```python
from build123d import *

# Parameters (mm, degrees)
BOSS_EXTRUDE1_DEPTH = 12.7
SKETCH2_R           = 3.175
CUT_EXTRUDE1_DEPTH  = 223.159267194


with BuildPart() as part:
    # Sketch1 → Boss-Extrude1 (new body)
    with BuildSketch(Plane(origin=(0, 0, 0), x_dir=(1, 0, 0), z_dir=(0, 1, 0))):
        with BuildLine():
            Line((-88.9, -25.4), (-71.842048969, -25.4))
            ThreePointArc((-71.842048969, -25.4), (0, -76.2), (71.842048969, -25.4))
            Line((71.842048969, -25.4), (88.9, -25.4))
            Line((88.9, -25.4), (88.9, -203.2))
            Line((88.9, -203.2), (-88.9, -203.2))
            Line((-88.9, -203.2), (-88.9, -25.4))
        make_face()
    extrude(amount=BOSS_EXTRUDE1_DEPTH)

    # Sketch2 → Cut-Extrude1 (cut, through all)
    with BuildSketch(Plane(origin=(0, 12.7, 0), x_dir=(1, 0, 0), z_dir=(0, 1, 0))):
        with Locations(Location((-19.05, -184.15, 0), (0, 0, 270))):
            Circle(SKETCH2_R)
        with Locations(Location((19.05, -184.15, 0), (0, 0, 270))):
            Circle(SKETCH2_R)
        with Locations(Location((57.15, -184.15, 0), (0, 0, 270))):
            Circle(SKETCH2_R)
        with Locations(Location((-57.15, -184.15, 0), (0, 0, 270))):
            Circle(SKETCH2_R)
    extrude(amount=-CUT_EXTRUDE1_DEPTH, mode=Mode.SUBTRACT)


solid = part.part
```
Input: part model. Units: mm. Frame: model coordinates. Give positions to 0.01 mm unless a question says otherwise; leave off trailing zeros. Loops run counter-clockwise (first coordinate to the right, second up) from the corner with the lowest first, then second, coordinate; pieces in that order, holes last. Notation, with made-up numbers: M 82.25,3 L 130.25,3 A14 cw 130.25,14 Z; hole C 71,-34 d9. An arc over 180 degrees is marked long. Answer as CSV lines item,"result". Start each with the question number.
1. Section C-C on y = 3.75. Return loops of the section in (x, z) (3 decimals), plus the area to 3 significant figures.
2. Pull-direction query (X, two-part tool) for faces 1 (the face through (88.9, 6, 113)), 2 (the face through (55.93, 6.44, 187.08)), 3 (the face through (-88.9, 6, 116)); classes: released by +X, released by -X, zero draft, split by the parting line, or undercut.
3. Section A-A on z = 184.15. Return loops of the section in (x, y) (3 decimals), plus the area to 3 significant figures.
4. Section B-B on x = 19.05. Return loops of the section in (y, z) (3 decimals), plus the area to 3 significant figures.
5. Pin query (flat end, axial travel): P1, Ø8.5, axis at x = -57.15, z = 184.15, coming from the -Y side; P2, Ø1, axis at x = -33, y = 4, coming from the -Z side. Return the tip coordinate at first contact, or that it passes through.
6. Section D-D on z = 69. Return loops of the section in (x, y).
7. Line query: L1, parallel to X at y = 6, z = 184.15 (3 decimals); L2, parallel to Z at x = -56.5, y = 12; L3, parallel to X at y = 5, z = 51. Output: solid intervals per line, ascending.
Computed values:
1,outline,"M -88.9,25.4 L -71.842,25.4 A76.2 cw 71.842,25.4 L 88.9,25.4 L 88.9,203.2 L -88.9,203.2 Z; hole C -57.15,184.15 d6.35; hole C -19.05,184.15 d6.35; hole C 19.05,184.15 d6.35; hole C 57.15,184.15 d6.35"
1,area,"26,200 mm²"
2,face 1,"released by +X"
2,face 2,"undercut"
2,face 3,"released by -X"
3,outline,"M -88.9,0 L -60.325,0 L -60.325,12.7 L -88.9,12.7 Z; M -53.975,0 L -22.225,0 L -22.225,12.7 L -53.975,12.7 Z; M -15.875,0 L 15.875,0 L 15.875,12.7 L -15.875,12.7 Z; M 22.225,0 L 53.975,0 L 53.975,12.7 L 22.225,12.7 Z; M 60.325,0 L 88.9,0 L 88.9,12.7 L 60.325,12.7 Z"
3,area,"1,940 mm²"
4,outline,"M 0,73.78 L 12.7,73.78 L 12.7,180.975 L 0,180.975 Z; M 0,187.325 L 12.7,187.325 L 12.7,203.2 L 0,203.2 Z"
4,area,"1,560 mm²"
5,P1,"stops at y = 0"
5,P2,"stops at z = 68.44"
6,outline,"M -88.9,0 L -32.33,0 L -32.33,12.7 L -88.9,12.7 Z; M 32.33,0 L 88.9,0 L 88.9,12.7 L 32.33,12.7 Z"
7,L1,"x = -88.9 to -60.325, -53.975 to -22.225, -15.875 to 15.875, 22.225 to 53.975, 60.325 to 88.9"
7,L2,"z = 51.13 to 181.04, 187.26 to 203.2"
7,L3,"x = -88.9 to -56.62, 56.62 to 88.9"
